Source: CAD feature listing. Evaluate the final solid. Frame: model axes, mm. A direction names the side the tool comes from. Round coordinates to 2 decimals unless told otherwise and drop trailing zeros. Write each loop counter-clockwise with the first axis right and the second up, starting at its lowest first coordinate (ties: lowest second). Pieces come first, ordered by that corner, then holes. Notation, with made-up numbers: (-6, 14.25) -> (31, 14.25) arc R25 cw to (31, 43.25) -> close; hole circle Ø1 at (79, 46.5). An arc over 180 degrees is marked (long way). Return JSON: item names as keys, results as strings. Group by question number.
from build123d import *

# Parameters (mm, degrees)
F0_W      = 46.2
F0_H      = 46.2
F1_DEPTH  = 1.5
F2_W      = 46.2
F2_H      = 46.2
F2_R      = 21.5
F3_DEPTH  = 27
F4_R      = 6.2
F4_R_2    = 1.5
F5_DEPTH  = 6
F6_R      = 6.2
F6_R_2    = 4.6
F7_DEPTH  = 9
F9_DEPTH  = 13.2
F11_DEPTH = 3.1894764338
F12_W     = 12
F12_H     = 15
F13_DEPTH = 11
F15_DEPTH = 9


with BuildPart() as f1:
    # F0 (on Top) → F1 (new body)
    with BuildSketch(Plane.XY):
        with Locations((23.1, 23.1)):
            Rectangle(F0_W, F0_H)
    extrude(amount=F1_DEPTH)

    # F2 (on face) → F3 (join)
    with BuildSketch(Plane.XY.offset(1.5)):
        with Locations((23.1, 23.1)):
            Rectangle(F2_W, F2_H)
        with Locations((23.1, 23.1)):
            Circle(F2_R, mode=Mode.SUBTRACT)
    extrude(amount=F3_DEPTH)

    # F4 (on face) → F5 (join)
    with BuildSketch(Plane.XY.offset(1.5)):
        with Locations((23.1, 23.1)):
            Circle(F4_R)
        with Locations((23.1, 23.1)):
            Circle(F4_R_2, mode=Mode.SUBTRACT)
    extrude(amount=F5_DEPTH)

    # F6 (on face) → F7 (join)
    with BuildSketch(Plane.XY.offset(7.5)):
        with Locations((23.1, 23.1)):
            Circle(F6_R)
        with Locations((23.1, 23.1)):
            Circle(F6_R_2, mode=Mode.SUBTRACT)
    extrude(amount=F7_DEPTH)

    # F8 (on face) → F9 (join)
    with BuildSketch(Plane.XY.offset(1.5)):
        with BuildLine():
            ThreePointArc((3.9363687534, 28.8232191506), (3.1, 23.1), (3.9363687534, 17.3767808494))
            Line((3.9363687534, 17.3767808494), (9.3430104109, 17.3767808494))
            ThreePointArc((9.3430104109, 17.3767808494), (8.2, 23.1), (9.3430104109, 28.8232191506))
            Line((9.3430104109, 28.8232191506), (3.9363687534, 28.8232191506))
        make_face()
        with BuildLine():
            ThreePointArc((42.2636312466, 17.3767808494), (43.1, 23.1), (42.2636312466, 28.8232191506))
            Line((42.2636312466, 28.8232191506), (36.8569895891, 28.8232191506))
            ThreePointArc((36.8569895891, 28.8232191506), (38, 23.1), (36.8569895891, 17.3767808494))
            Line((36.8569895891, 17.3767808494), (42.2636312466, 17.3767808494))
        make_face()
    extrude(amount=F9_DEPTH)

    # F10 (on face) → F11 (cut, up to face)
    with BuildSketch(Plane(origin=(0, 46.2, 0), x_dir=(-1, 0, 0), z_dir=(0, 1, 0))):
        with BuildLine():
            ThreePointArc((-24.1, 11.3989794856), (-23.1, 1.5), (-22.1, 11.3989794856))
            ThreePointArc((-22.1, 11.3989794856), (-23.1, 12.3989794856), (-24.1, 11.3989794856))
        make_face()
    extrude(amount=-F11_DEPTH, mode=Mode.SUBTRACT)

    # F12 (on face) → F13 (cut)
    with BuildSketch(Plane.XY.offset(1.5)):
        with Locations((23.1, 37.1)):
            Rectangle(F12_W, F12_H)
    extrude(amount=F13_DEPTH, mode=Mode.SUBTRACT)

    # F14 (on face) → F15 (join)
    with BuildSketch(Plane.XY.offset(1.5)):
        with BuildLine():
            Line((17.1, 40.6), (17.1, 43.7458228221))
            ThreePointArc((17.1, 43.7458228221), (16.2947624154, 43.4945762745), (15.5, 43.2119367541))
            Line((15.5, 43.2119367541), (15.5, 40.6))
            Line((15.5, 40.6), (17.1, 40.6))
        make_face()
        with BuildLine():
            ThreePointArc((30.7, 43.2119367541), (29.9052375846, 43.4945762745), (29.1, 43.7458228221))
            Line((29.1, 43.7458228221), (29.1, 32.6))
            Line((29.1, 32.6), (30.7, 32.6))
            Line((30.7, 32.6), (30.7, 43.2119367541))
        make_face()
    extrude(amount=F15_DEPTH)


solid = f1.part
Item 1: Cut plane B-B on y = 23.1. Output: boundary loops of the cut face in (x, z).
Item 2: Cut plane C-C on z = 21.5. Output: boundary loops of the cut face in (x, y), and give its area (3 significant figures).
Item 3: Material intervals for probe 1 along Y at (x, z) = (23.1, 14); probe 2 along X at (y, z) = (23.1, 20.5), sorted ascending.
Item 4: First-contact query: pin 1 Ø0.5 at (x, y) = (16, 41.5) entering from +Z; pin 2 Ø3.5 at (x, y) = (22.5, 22.5) entering from +Z; pin 3 Ø8 at (x, z) = (23.1, 6.5) entering from +Y. Flat tips, straight axial feed; report the tip coordinate or a pass-through.
Item 5: Pull-direction query (Z, two-part tool) for faces 1 (the cylindrical face through (21.6, 23.17, 4.46)), 2 (the flat face through (22, 44.6, 12)), 3 (the flat face through (16, 42, 10.5)); classes: +Z half, -Z half, draft (parallel to the pull), parting line (faces both ways), or undercut.
Item 6: Cut plane D-D on x = 11. Output: boundary loops of the cut face in (y, z).
Item 7: Set-up query: faces 4 (the flat face through (23, 0, 14)), 5 (the cylindrical face through (43.1, 23, 8)), 6 (the cylindrical face through (23.306, 45.411, 1.504)). Return all of +Z, -Z, +X, -X, +Y, -Y with unobstructed straight access to the full face (end or side cutting, diameter ignored); none if empty.
Item 8: Cut plane A-A on z = 6.5. Output: boundary loops of the cut face in (x, y), and give its area (3 significant figures).
Here are the results:
{
 "1": {"outline": "(0, 0) -> (46.2, 0) -> (46.2, 28.5) -> (44.6, 28.5) -> (44.6, 1.5) -> (43.1, 1.5) -> (43.1, 14.7) -> (38, 14.7) -> (38, 1.5) -> (29.3, 1.5) -> (29.3, 16.5) -> (27.7, 16.5) -> (27.7, 7.5) -> (24.6, 7.5) -> (24.6, 1.5) -> (21.6, 1.5) -> (21.6, 7.5) -> (18.5, 7.5) -> (18.5, 16.5) -> (16.9, 16.5) -> (16.9, 1.5) -> (8.2, 1.5) -> (8.2, 14.7) -> (3.1, 14.7) -> (3.1, 1.5) -> (1.6, 1.5) -> (1.6, 28.5) -> (0, 28.5) -> close"},
 "2": {"outline": "(0, 0) -> (46.2, 0) -> (46.2, 46.2) -> (0, 46.2) -> close; hole circle Ø43 at (23.1, 23.1)", "area": "682 mm^2"},
 "3": {"probe 1": "y = 0 to 1.6, 16.9 to 18.5, 27.7 to 29.3, 44.6 to 46.2", "probe 2": "x = 0 to 1.6, 44.6 to 46.2"},
 "4": {"pin 1": "stops at z = 10.5", "pin 2": "stops at z = 7.5", "pin 3": "stops at y = 29.3"},
 "5": {"face 1": "draft", "face 2": "undercut", "face 3": "+Z half"},
 "6": {"outline": "(0, 0) -> (46.2, 0) -> (46.2, 28.5) -> (40.87, 28.5) -> (40.87, 1.5) -> (5.33, 1.5) -> (5.33, 28.5) -> (0, 28.5) -> close"},
 "7": {"face 4": "+Z, -Z, +X, -X, -Y", "face 5": "+Z", "face 6": "+Y"},
 "8": {"outline": "(0, 0) -> (46.2, 0) -> (46.2, 46.2) -> (28.1, 46.2) -> (28.1, 44.6) -> (29.1, 44.6) -> (29.1, 32.6) -> (30.7, 32.6) -> (30.7, 43.21) arc R21.5 cw (long way) to (15.5, 43.21) -> (15.5, 40.6) -> (17.1, 40.6) -> (17.1, 44.6) -> (18.1, 44.6) -> (18.1, 46.2) -> (0, 46.2) -> close; (3.94, 17.38) -> (9.34, 17.38) arc R14.9 cw to (9.34, 28.82) -> (3.94, 28.82) arc R20 ccw to start; circle Ø12.4 at (23.1, 23.1); (36.86, 17.38) -> (42.26, 17.38) arc R20 ccw to (42.26, 28.82) -> (36.86, 28.82) arc R14.9 cw to start; hole circle Ø3 at (23.1, 23.1)", "area": "918 mm^2"}
}
